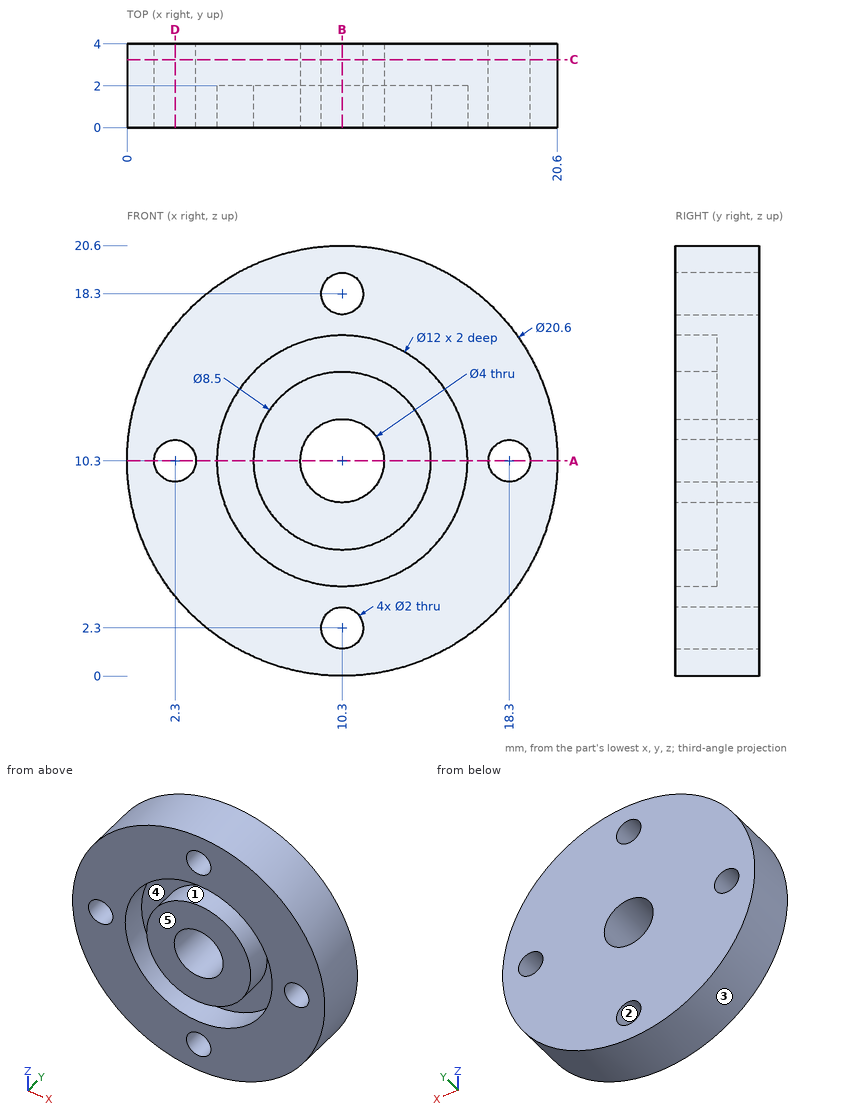
Part print with two shaded views. Sizes in mm from the minimum x, y, z corner. A direction names the side the tool comes from. Coordinates: 2 decimals unless noted, no trailing zeros. Write each loop counter-clockwise with the first axis right and the second up, starting at its lowest first coordinate (ties: lowest second). Pieces come first, ordered by that corner, then holes. Notation, with made-up numbers: (4.25, 67) - (42.25, 67) arc R21 ccw to (42.25, 72) - close; hole circle Ø10 at (8.25, 81). An arc over 180 degrees is marked (long way). Put each result on its own line as item: value.
1. Two-plate mould, pull along Z, no slides. Class the marked faces 3, 4 and 5: +Z half, -Z half, draft (parallel to the pull), parting line (faces both ways), or undercut.
Final values:
face 3: parting line
face 4: undercut
face 5: draft
2. Band-saw the part on D-D (x = 2.3). Write the cut outline in (y, z).
Final values:
outline: (0, 3.81) - (4, 3.81) - (4, 9.3) - (0, 9.3) - close; (0, 11.3) - (4, 11.3) - (4, 16.79) - (0, 16.79) - close
3. Flat gauge pin, fed straight in: pin 1 Ø1 at (y, z) = (1.5, 18) entering from +X. Where does the tip first touch, or does it go through?
Final values:
pin 1: stops at x = 17.67
4. Band-saw the part on C-C (y = 3.25). Write the cut outline in (x, z), then the cut area to 3 significant figures.
Final values:
outline: circle Ø20.6 at (10.3, 10.3); hole circle Ø2 at (2.3, 10.3); hole circle Ø4 at (10.3, 10.3); hole circle Ø2 at (10.3, 2.3); hole circle Ø2 at (10.3, 18.3); hole circle Ø2 at (18.3, 10.3)
area: 308 mm²
5. Probe line 1 along X through (y, z) = (0.85, 10.3); line 2 along Z through (x, y) = (12.75, 1.1); line 3 along Z through (x, y) = (8.5, 0.45). List the from-to ranges inside material, lowest first. Write a range as [from, to].
Final values:
line 1: x = [0, 1.3], [3.3, 4.3], [6.05, 8.3], [12.3, 14.55], [16.3, 17.3], [19.3, 20.6]
line 2: z = [0.3, 4.82], [6.83, 13.77], [15.78, 20.3]
line 3: z = [0.16, 4.58], [6.45, 9.43], [11.17, 14.15], [16.02, 20.44]
6. Band-saw the part on A-A (z = 10.3). Write the cut outline in (x, y), then the cut area to 3 significant figures.
Final values:
outline: (0, 0) - (1.3, 0) - (1.3, 4) - (0, 4) - close; (3.3, 0) - (4.3, 0) - (4.3, 2) - (6.05, 2) - (6.05, 0) - (8.3, 0) - (8.3, 4) - (3.3, 4) - close; (12.3, 0) - (14.55, 0) - (14.55, 2) - (16.3, 2) - (16.3, 0) - (17.3, 0) - (17.3, 4) - (12.3, 4) - close; (19.3, 0) - (20.6, 0) - (20.6, 4) - (19.3, 4) - close
area: 43.4 mm²
7. Band-saw the part on B-B (x = 10.3). Write the cut outline in (y, z).
Final values:
outline: (0, 0) - (4, 0) - (4, 1.3) - (0, 1.3) - close; (0, 3.3) - (4, 3.3) - (4, 8.3) - (0, 8.3) - (0, 6.05) - (2, 6.05) - (2, 4.3) - (0, 4.3) - close; (0, 12.3) - (4, 12.3) - (4, 17.3) - (0, 17.3) - (0, 16.3) - (2, 16.3) - (2, 14.55) - (0, 14.55) - close; (0, 19.3) - (4, 19.3) - (4, 20.6) - (0, 20.6) - close
8. 3-axis set-ups, long thin cutter, end or side, ignore diameter. For the marked faces 1 and 2: which of +Z, -Z, +X, -X, +Y, -Y reach the whole face in a straight line?
Final values:
face 1: -Y
face 2: +Y, -Y
